Source: CAD feature listing. Evaluate the final solid. Frame: model axes, mm. A direction names the side the tool comes from. Round coordinates to 2 decimals unless told otherwise and drop trailing zeros. Write each loop counter-clockwise with the first axis right and the second up, starting at its lowest first coordinate (ties: lowest second). Pieces come first, ordered by that corner, then holes. Notation, with made-up numbers: M -4.75,7.5 L 48.25,7.5 A20 cw 48.25,40.5 Z; hole C 13.5,-33 d9. An arc over 180 degrees is marked long. Put each result on its own line as item: value. Start each with the question number.
```python
from build123d import *

# Parameters (mm, degrees)
BOSS_EXTRUDE1_DEPTH = 76.2


with BuildPart() as part:
    # Sketch1 → Boss-Extrude1 (new body)
    with BuildSketch(Plane.XY):
        with BuildLine():
            ThreePointArc((-263.258240929, -25.4), (-288.658240929, 0), (-263.258240929, 25.4))
            Line((-263.258240929, 25.4), (-250.558240929, 25.4))
            Line((-250.558240929, 25.4), (-250.558240929, 63.5))
            Line((-250.558240929, 63.5), (-263.217595671, 63.5))
            Line((-263.217595671, 63.5), (-263.258240929, 63.5))
            ThreePointArc((-263.258240929, 63.5), (-326.758240929, 0), (-263.258240929, -63.5))
            ThreePointArc((-263.258240929, -63.5), (-244.427108864, -60.643536054), (-227.290164194, -52.33113276))
            Line((-227.290164194, -52.33113276), (-248.871010235, -20.932453104))
            ThreePointArc((-248.871010235, -20.932453104), (-255.725788103, -24.257414422), (-263.258240929, -25.4))
        make_face()
    extrude(amount=BOSS_EXTRUDE1_DEPTH)


solid = part.part
```
(1) Pull-direction query (Y, two-part tool) for faces 3 (the flat face through (-237.93, -36.85, 37.57)), 4 (the flat face through (-289, 1, 0)), 5 (the flat face through (-257, 25.4, 38)); classes: +Y half, -Y half, draft (parallel to the pull), parting line (faces both ways), or undercut.
(2) Section query B-B (z = 14.5). Return loops of the section in (x, y).
(3) Contact query for flat-ended pins moving along their axis: P1, Ø8, axis at y = 21.5, z = 10, coming from the -X side; P2, Ø5, axis at x = -312, z = 64.5, coming from the -Y side; P3, Ø10, axis at y = 11, z = 55, coming from the +X side. Output: stop coordinate, or through.
(4) Access query for faces 1 (the flat face through (-250.558, 44, 38)), 2 (the flat face through (-257, 63.5, 38)). Directions: +Z, -Z, +X, -X, +Y, -Y. A direction counts if a zero-diameter tool reaches every point of the face in a straight line with its end or side. Return the directions, or none.
(5) Section query A-A (x = -276). Return loops of the section in (y, z), and give its area (3 significant figures).
(6) Ray query, line 1 along Y through (x, z) = (-257.5, 19); line 2 along Y through (x, z) = (-255, 69); line 3 along Y through (x, z) = (-318, 30.5). Return the intervals inside material, ascending.
(7) Section query D-D (x = -309.5). Return loops of the section in (y, z).
(8) Section query C-C (y = 0). Return loops of the section in (x, z).
Entries:
1. face 3: +Y half
1. face 4: draft
1. face 5: undercut
2. outline: M -263.26,25.4 L -250.56,25.4 L -250.56,63.5 L -263.26,63.5 A63.5 ccw long -227.29,-52.33 L -248.87,-20.93 A25.4 cw long Z
3. P1: x = -324.3
3. P2: y = -43.52
3. P3: x = -282.99
4. face 1: +Z, -Z, +X, +Y
4. face 2: +Z, -Z, +X, -X, +Y
5. outline: M -62.21,0 L -21.97,0 L -21.97,76.2 L -62.21,76.2 Z; M 21.97,0 L 62.21,0 L 62.21,76.2 L 21.97,76.2 Z
5. area: 6,130 mm2
6. line 1: -63.24 to -24.74, 25.4 to 63.5
6. line 2: -62.96 to -24.02, 25.4 to 63.5
6. line 3: -32.18 to 32.18
7. outline: M -43.52,0 L 43.52,0 L 43.52,76.2 L -43.52,76.2 Z
8. outline: M -326.76,0 L -288.66,0 L -288.66,76.2 L -326.76,76.2 Z
